Here's how the part is built. I have some questions about the finished solid (model axes, mm). A direction names the side the tool comes from. Coordinates: 2 decimals unless noted, no trailing zeros. Write each loop counter-clockwise with the first axis right and the second up, starting at its lowest first coordinate (ties: lowest second). Pieces come first, ordered by that corner, then holes.
Item 1: If we section it at A-A (z = 1): Please give me the cut outline in (x, y).
Item 2: We'd pull the mould along X, two halves only. Please class faces 4 (the face through (1.282, -2.262, 0.209)), 5 (the face through (0, 0, 0)), 6 (the face through (-1.282, 2.262, 0.209)): +X half, -X half, draft (parallel to the pull), parting line (faces both ways), or undercut.
Item 3: I'm going to push a flat-ended pin straight in: pin 1 Ø1.5 at (x, y) = (0.5, -0.5) entering from +Z. Where does the tip first touch, or does it pass through?
Item 4: For faces 1 (the face through (-1.5, 0.07, 7.6)), 2 (the face through (2, 0, 15)), 3 (the face through (-1.5, -0.07, -17.71)), which set-ups out of +Z, -Z, +X, -X, +Y, -Y let a thin tool reach every point of the face, with its end or its side?
Item 5: If we section it at B-B (y = 0): Please give me the cut outline in (x, z), then the cut area to 3 significant figures.
Item 6: If I drill on line 1 (Z direction, x = -2.1, y = 0.75); line 2 (Z direction, x = 0.1, y = 1); line 3 (Y direction, x = 0.15, z = -16), over which ranges is the centre line in solid material (lowest first)?
Item 7: If we section it at D-D (z = -18): Please give me the cut outline in (x, y).
Item 8: If we section it at C-C (z = -5.5): Please give me the cut outline in (x, y), then the cut area to 3 significant figures.
from build123d import *

# Parameters (mm, degrees)
PAD_DEPTH    = 15
SKETCH001_R  = 1.5
POCKET_DEPTH = 15
SKETCH002_R  = 1.5
PAD001_DEPTH = 5.5


with BuildPart() as body001:
    # Sketch003 → Revolution (revolve)
    with BuildSketch(Plane.YZ):
        Polygon((2, 15.5), (5, 15.5), (5, -15.5), (2, -15.5), (3.923501, -13.576499), (3.923501, 13.576499), align=None)
    revolve(axis=Axis((0, 0, 0), (0, 0, 1)))


with BuildPart() as cut:
    # Sketch → Pad (new body, symmetric)
    with BuildSketch(Plane.XY):
        Polygon((2.6, 1.501111), (0, 3.002221), (-2.6, 1.501111), (-2.6, -1.501111), (0, -3.002221), (2.6, -1.501111), align=None)
    extrude(amount=PAD_DEPTH, both=True)

    # Sketch001 (on Face8 of Pad) → Pocket (cut)
    with BuildSketch(Plane.XY.offset(15)):
        Circle(SKETCH001_R)
    extrude(amount=-POCKET_DEPTH, mode=Mode.SUBTRACT)

    # Sketch002 (on Face4 of Pocket) → Pad001 (join)
    with BuildSketch(Plane(origin=(0, 0, -15), x_dir=(1, 0, 0), z_dir=(0, 0, -1))):
        Circle(SKETCH002_R)
    extrude(amount=PAD001_DEPTH)

    # Cut: cut Body001
    add(body001.part, mode=Mode.SUBTRACT)


solid = cut.part
Answer list:
1. outline: (-2.6, -1.5) - (0, -3) - (2.6, -1.5) - (2.6, 1.5) - (0, 3) - (-2.6, 1.5) - close; hole circle Ø3 at (0, 0)
2. face 4: +X half
2. face 5: undercut
2. face 6: -X half
3. pin 1: stops at z = 0
4. face 1: +Z
4. face 2: +Z, +X, -X, +Y, -Y
4. face 3: -Z
5. outline: (-2.6, -14.9) - (-2.5, -15) - (-1.5, -15) - (-1.5, -20.5) - (1.5, -20.5) - (1.5, -15) - (2.5, -15) - (2.6, -14.9) - (2.6, 14.9) - (2.5, 15) - (1.5, 15) - (1.5, 0) - (-1.5, 0) - (-1.5, 15) - (-2.5, 15) - (-2.6, 14.9) - close
5. area: 127 mm2
6. line 1: z = -15 to 15
6. line 2: z = -20.5 to 0
6. line 3: y = -1.49 to 1.49
7. outline: circle Ø3 at (0, 0)
8. outline: (-2.6, -1.5) - (0, -3) - (2.6, -1.5) - (2.6, 1.5) - (0, 3) - (-2.6, 1.5) - close
8. area: 23.4 mm2
